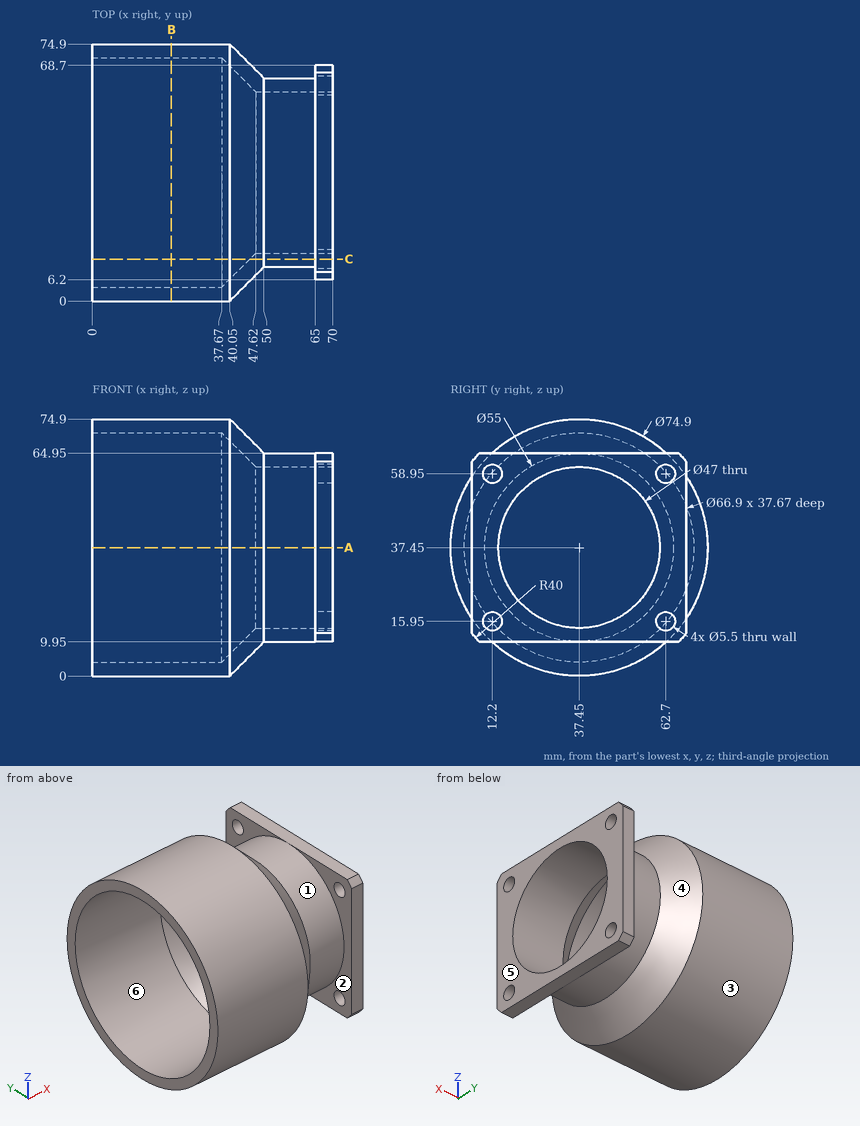
Job drawing, mm, ordinate dimensions from the low corner. One solid piece. A direction names the side the tool comes from. Round coordinates to 2 decimals unless told otherwise and drop trailing zeros. Loops run counter-clockwise (first coordinate to the right, second up) from the corner with the lowest first, then second, coordinate; pieces in that order, holes last.
Item 1: Cut at B-B, the plane x = 23. Give the cut face in (y, z), then the cut area to 3 significant figures.
Item 2: 3-axis set-ups, long thin cutter, end or side, ignore diameter. For the marked faces 1, 2 and 3: which of +Z, -Z, +X, -X, +Y, -Y reach the whole face in a straight line?
Item 3: Drill centre lines: line 1 (Y direction, x = 58, z = 37.45); line 2 (Y direction, x = 22.5, z = 37.45); line 3 (Z direction, x = 66, y = 62). Where is each one in solid material? Low to high.
Item 4: Mould opens along Y. For the marked faces 4, 5 and 6 say: +Y half, -Y half, draft (parallel to the pull), parting line (faces both ways), or undercut.
Item 5: Cut at A-A, the plane z = 37.45. Give the cut face in (x, y), then the cut area to 3 significant figures.
Item 6: Cut at C-C, the plane y = 12.2. State how many separate pieces and enclosed holes the cut face has, then the cut area to 3 significant figures.
Item 7: Drop flat-ended pins along their axis: P1, Ø12, axis at y = 32, z = 48, coming from the +X side; P2, Ø12, axis at x = 37, y = 37.5, coming from the +Z side; P3, Ø3.5, axis at y = 62.7, z = 15.95, coming from the +X side (1 decimal); P4, Ø8, axis at x = 29, y = 11.5, coming from the +Z side. Give the stop position or say it passes through.
A:
1. outline: circle Ø74.9 at (37.45, 37.45); hole circle Ø66.9 at (37.45, 37.45)
1. area: 891 mm2
2. face 1: none
2. face 2: -Y
2. face 3: -X
3. line 1: y = 9.95 to 13.95, 60.95 to 64.95
3. line 2: y = 0 to 4, 70.9 to 74.9
3. line 3: z = 9.95 to 13.29, 18.61 to 56.29, 61.61 to 64.95
4. face 4: parting line
4. face 5: draft
4. face 6: undercut
5. outline: (0, 0) - (40.05, 0) - (50, 9.95) - (65, 9.95) - (65, 6.2) - (70, 6.2) - (70, 13.95) - (47.62, 13.95) - (37.67, 4) - (0, 4) - close; (0, 70.9) - (37.67, 70.9) - (47.62, 60.95) - (70, 60.95) - (70, 68.7) - (65, 68.7) - (65, 64.95) - (50, 64.95) - (40.05, 74.9) - (0, 74.9) - close
5. area: 645 mm2
6. separate pieces: 3
6. enclosed holes: 0
6. area: 1,280 mm2
7. P1: passes through
7. P2: stops at z = 74.9
7. P3: stops at x = 46.1
7. P4: stops at z = 67.79
